Could you check a few things on this model? Use its own coordinates, in mm. A direction names the side the tool comes from. Round coordinates to 2 decimals unless told otherwise and drop trailing zeros. Order: outer loops, then holes, each group sorted by start corner. A loop starts at its lowest first (then second) coordinate and runs counter-clockwise, first axis right, second up. Notation, with made-up numbers: (46, 54.25) -> (60, 54.25) arc R23 ccw to (60, 69.25) -> close; hole circle Ø8 at (54.25, 7.25). An arc over 180 degrees is marked (long way). One line per question, with ' | ' between items.
```python
from build123d import *

# Parameters (mm, degrees)
SKETCH_1_W          = 20
SKETCH_1_H          = 12
EXTRUDE_1_DEPTH     = 2
EXTRUDE_2_DEPTH     = 6
SKETCH_5_R          = 0.5
CUT_EXTRUDE_1_DEPTH = 25.657656012
SKETCH_5_3_R        = 1
CUT_EXTRUDE_2_DEPTH = 1
SKETCH_6_R          = 0.4
CUT_EXTRUDE_3_DEPTH = 25.657656012


with BuildPart() as part:
    # 草图1 → 凸台-拉伸1 (new body)
    with BuildSketch(Plane(origin=(0, 0, 0), x_dir=(1, 0, 0), z_dir=(0, 1, 0))):
        with Locations((10, 6)):
            Rectangle(SKETCH_1_W, SKETCH_1_H)
    extrude(amount=EXTRUDE_1_DEPTH)

    # 草图4 → 凸台-拉伸2 (add)
    with BuildSketch(Plane(origin=(0, 2, 0), x_dir=(1, 0, 0), z_dir=(0, 1, 0))):
        with BuildLine():
            Line((5, 11.75), (5, 12))
            Line((5, 12), (0, 12))
            Line((0, 12), (0, 8.839454173))
            ThreePointArc((0, 8.839454173), (2.107281684, 10.969374281), (5, 11.75))
        make_face()
        with BuildLine():
            Line((5, 0), (5, 0.25))
            ThreePointArc((5, 0.25), (2.107281684, 1.030625719), (0, 3.160545827))
            Line((0, 3.160545827), (0, 0))
            Line((0, 0), (5, 0))
        make_face()
        with BuildLine():
            Line((20, 12), (15, 12))
            Line((15, 12), (15, 11.75))
            ThreePointArc((15, 11.75), (17.892718316, 10.969374281), (20, 8.839454173))
            Line((20, 8.839454173), (20, 12))
        make_face()
        with BuildLine():
            ThreePointArc((20, 3.160545827), (17.892718316, 1.030625719), (15, 0.25))
            Line((15, 0.25), (15, 0))
            Line((15, 0), (20, 0))
            Line((20, 0), (20, 3.160545827))
        make_face()
    extrude(amount=EXTRUDE_2_DEPTH)

    # 草图5 → 切除-拉伸1 (cut, through all)
    with BuildSketch(Plane.XZ):
        with Locations(Location((10, -1.2, 0), (0, 0, 270))):
            Circle(SKETCH_5_R)
        with Locations(Location((10, -10.8, 0), (0, 0, 270))):
            Circle(SKETCH_5_R)
    extrude(amount=-CUT_EXTRUDE_1_DEPTH, mode=Mode.SUBTRACT)

    # 草图5<3> → 切除-拉伸2 (cut)
    with BuildSketch(Plane.XZ):
        with Locations(Location((10, -1.2, 0), (0, 0, 270))):
            Circle(SKETCH_5_3_R)
        with Locations(Location((10, -10.8, 0), (0, 0, 270))):
            Circle(SKETCH_5_3_R)
    extrude(amount=-CUT_EXTRUDE_2_DEPTH, mode=Mode.SUBTRACT)

    # 草图6 → 切除-拉伸3 (cut, through all)
    with BuildSketch(Plane.XZ):
        with Locations(Location((3, -3, 0), (0, 0, 270))):
            Circle(SKETCH_6_R)
        with Locations(Location((3, -9, 0), (0, 0, 270))):
            Circle(SKETCH_6_R)
        with Locations(Location((7, -9, 0), (0, 0, 270))):
            Circle(SKETCH_6_R)
        with Locations(Location((7, -3, 0), (0, 0, 270))):
            Circle(SKETCH_6_R)
    extrude(amount=-CUT_EXTRUDE_3_DEPTH, mode=Mode.SUBTRACT)


solid = part.part
```
1. I want a section at C-C on z = -1.2. List the corners of the cut face in (x, y) for me.
From the geometry:
outline: (0, 0) -> (9, 0) -> (9, 1) -> (9.5, 1) -> (9.5, 2) -> (1.83, 2) -> (1.83, 8) -> (0, 8) -> close; (10.5, 1) -> (11, 1) -> (11, 0) -> (20, 0) -> (20, 8) -> (18.17, 8) -> (18.17, 2) -> (10.5, 2) -> close
2. I need wall thicknesses on probe 1 along X at (y, z) = (0.6, -10.8); probe 2 along Z at (x, y) = (10.75, 0.5); probe 3 along Y at (x, z) = (18.5, -3.75). Which ranges of each line are inside material? Lowest first, please.
From the geometry:
probe 1: x = 0 to 9, 11 to 20 | probe 2: z = -12 to -11.46, -10.14 to -1.86, -0.54 to 0 | probe 3: y = 0 to 2
3. If we mould it in two halves opening along X, with no side actions, what happens to faces 1 (the face through (0, 1, -6)), 2 (the face through (2.071, 4.958, -10.948)), 3 (the face through (10, 2, -6)), 4 (the face through (20, 1, -6))? For each: pulls with the +X half, pulls with the -X half, needs draft (parallel to the pull), parting line crosses it, or undercut.
From the geometry:
face 1: pulls with the -X half | face 2: undercut | face 3: undercut | face 4: pulls with the +X half
4. I'm going to push a flat-ended pin straight in: pin 1 (5 mm diameter, centred on x = 13.5, z = -4.5, fed in from +Y). Where does the tip first touch, or does it pass through?
From the geometry:
pin 1: stops at y = 2
5. On a 3-axis mill with a long thin cutter (end or side, diameter ignored), from which of +Z, -Z, +X, -X, +Y, -Y can I reach the whole of each face in a straight line? I mean faces 5 (the face through (10, 1, -12)), 6 (the face through (10, 1, -10)), 7 (the face through (2.14, 4.96, -1.01)). Say none if no direction works.
From the geometry:
face 5: -Z, +X, -X, +Y, -Y | face 6: -Y | face 7: +Y
6. I want a section at D-D on z = -4. List the corners of the cut face in (x, y) for me, and give its area (3 significant figures).
From the geometry:
outline: (0, 0) -> (20, 0) -> (20, 2) -> (0, 2) -> close | area: 40.0 mm²
7. I want a section at B-B on x = 7. List the corners of the cut face in (y, z) for me, and give its area (3 significant figures).
From the geometry:
outline: (0, -12) -> (2, -12) -> (2, -9.4) -> (0, -9.4) -> close; (0, -8.6) -> (2, -8.6) -> (2, -3.4) -> (0, -3.4) -> close; (0, -2.6) -> (2, -2.6) -> (2, 0) -> (0, 0) -> close | area: 20.8 mm²
8. I want a section at A-A on y = 5.25. List the corners of the cut face in (x, z) for me.
From the geometry:
outline: (0, -12) -> (5, -12) -> (5, -11.75) arc R5.75 cw to (0, -8.84) -> close; (0, -3.16) arc R5.75 cw to (5, -0.25) -> (5, 0) -> (0, 0) -> close; (15, -12) -> (20, -12) -> (20, -8.84) arc R5.75 cw to (15, -11.75) -> close; (15, -0.25) arc R5.75 cw to (20, -3.16) -> (20, 0) -> (15, 0) -> close
